from build123d import *

# Parameters (mm, degrees)
F0_W     = 35
F0_H     = 50
F1_DEPTH = 10
F2_R     = 2.5
F3_DEPTH = 10.001
F4_R     = 2.5
F5_DEPTH = 25
F7_DEPTH = 25
F8_R     = 4.5
F9_DEPTH = 5.5


with BuildPart() as f1:
    # F0 (on Front) → F1 (new body)
    with BuildSketch(Plane.XZ):
        with Locations((17.5, 25)):
            Rectangle(F0_W, F0_H)
    extrude(amount=-F1_DEPTH)

    # F2 (on face) → F3 (cut, through all)
    with BuildSketch(Plane.XZ):
        with Locations((28, 6)):
            Circle(F2_R)
        with Locations((7, 23)):
            Circle(F2_R)
    extrude(amount=-F3_DEPTH, mode=Mode.SUBTRACT)

    # F4 (on face) → F5 (cut)
    with BuildSketch(Plane.XZ):
        with Locations((17.5, 25)):
            Circle(F4_R)
        with Locations((4.064971, 30.564971)):
            Circle(F4_R)
        with Locations((30.935029, 30.564971)):
            Circle(F4_R)
    extrude(amount=-F5_DEPTH, mode=Mode.SUBTRACT)

    # F6 (on face) → F7 (cut)
    with BuildSketch(Plane.XZ):
        with BuildLine():
            Line((0, 36), (10.358572, 36))
            ThreePointArc((10.358572, 36), (17.5, 33), (24.641428, 36))
            Line((24.641428, 36), (35, 36))
            Line((35, 36), (35, 50))
            Line((35, 50), (0, 50))
            Line((0, 50), (0, 36))
        make_face()
    extrude(amount=-F7_DEPTH, mode=Mode.SUBTRACT)

    # F8 (on face) → F9 (cut)
    with BuildSketch(Plane.XZ):
        with Locations((7, 23)):
            Circle(F8_R)
    extrude(amount=-F9_DEPTH, mode=Mode.SUBTRACT)


solid = f1.part
Source: CAD feature listing. Evaluate the final solid. Frame: model axes, mm. A direction names the side the tool comes from. Round coordinates to 2 decimals unless told otherwise and drop trailing zeros. Loops run counter-clockwise (first coordinate to the right, second up) from the corner with the lowest first, then second, coordinate; pieces in that order, holes last. Notation, with made-up numbers: (6.25, 27.25) - (50.25, 27.25) arc R30 ccw to (50.25, 63.25) - close; hole circle Ø10 at (-10.75, -11). An arc over 180 degrees is marked (long way). Write item = value, one per line. Start each with the question number.
Item 1: Section query D-D on z = 32.5. Output: boundary loops of the cut face in (x, y), plus the area to 3 significant figures.
Item 2: Section query C-C on y = 2.5. Output: boundary loops of the cut face in (x, z), plus the area to 3 significant figures.
Item 3: Reachability of faces 4 (the face through (33.244, 4.93, 29.607)), 5 (the face through (9, 5.5, 21)) from +Z, -Z, +X, -X, +Y, -Y: full face, straight path, thin tool, end or side. Return the list, or none.
Item 4: Section query B-B on x = 17.5. Output: boundary loops of the cut face in (y, z), plus the area to 3 significant figures.
Item 5: Mould query, pull axis X, two halves, no side actions, for faces 1 (the face through (0, 5, 18)), 2 (the face through (6.41, 2.71, 27.46)), 3 (the face through (17, 10, 18)). Classes: released by +X, released by -X, zero draft, split by the parting line, or undercut.
Item 6: Material intervals for line 1 (Z direction, x = 17.5, y = 5); line 2 (Z direction, x = 28, y = 3.5); line 3 (X direction, y = 8, z = 26), sorted ascending.
Item 7: Section query A-A on z = 6. Output: boundary loops of the cut face in (x, y).
Results list:
q1.outline = (0, 0) - (2.48, 0) - (2.48, 10) - (0, 10) - close; (5.65, 0) - (29.35, 0) - (29.35, 10) - (5.65, 10) - close; (32.52, 0) - (35, 0) - (35, 10) - (32.52, 10) - close
q1.area = 287 mm²
q2.outline = (0, 0) - (35, 0) - (35, 36) - (24.64, 36) arc R10 cw to (10.36, 36) - (0, 36) - close; hole circle Ø5 at (4.06, 30.56); hole circle Ø9 at (7, 23); hole circle Ø5 at (17.5, 25); hole circle Ø5 at (28, 6); hole circle Ø5 at (30.94, 30.56)
q2.area = 1,090 mm²
q3.face_4 = +Y, -Y
q3.face_5 = -Y
q4.outline = (0, 0) - (10, 0) - (10, 22.5) - (0, 22.5) - close; (0, 27.5) - (10, 27.5) - (10, 33) - (0, 33) - close
q4.area = 280 mm²
q5.face_1 = released by -X
q5.face_2 = undercut
q5.face_3 = zero draft
q6.line_1 = 0 to 22.5, 27.5 to 33
q6.line_2 = 0 to 3.5, 8.5 to 36
q6.line_3 = 0 to 15.21, 19.79 to 35
q7.outline = (0, 0) - (25.5, 0) - (25.5, 10) - (0, 10) - close; (30.5, 0) - (35, 0) - (35, 10) - (30.5, 10) - close
